Part model, mm, in its own coordinate system. A direction names the side the tool comes from. Give positions to 0.01 mm unless a question says otherwise; leave off trailing zeros. Order: outer loops, then holes, each group sorted by start corner. A loop starts at its lowest first (then second) coordinate and runs counter-clockwise, first axis right, second up. Notation, with made-up numbers: M 1,-6 L 32,-6 A17 ccw 32,-1 Z; hole C -14.75,3.25 d2. An arc over 180 degrees is marked long. Write each question's results on one line, items separated by ' | '. Start each with the question number.
from build123d import *

# Parameters (mm, degrees)
F1_DEPTH = 2540


with BuildPart() as f1:
    # F0 (on Front) → F1 (new body)
    with BuildSketch(Plane.XZ):
        with BuildLine():
            Line((153.9936810732, 85.9075784683), (30.2082335464, 16.8963483059))
            ThreePointArc((30.2082335464, 16.8963483059), (33.4933271093, 8.7304638603), (34.6124827204, 0))
            ThreePointArc((34.6124827204, 0), (33.5294597887, -8.5906511012), (30.3481664655, -16.6437000769))
            Line((30.3481664655, -16.6437000769), (153.9936810732, -85.7974737883))
            Line((153.9936810732, -85.7974737883), (153.9936810732, 85.9075784683))
        make_face()
        with BuildLine():
            ThreePointArc((30.2082335464, 16.8963483059), (0.1433871846, 34.6121857181), (-30.0672068078, 17.1460501237))
            Line((-30.0672068078, 17.1460501237), (0.2459637966, 0.192178832))
            Line((0.2459637966, 0.192178832), (30.2082335464, 16.8963483059))
        make_face()
        with BuildLine():
            Line((30.3481664655, -16.6437000769), (0.2459637966, 0.192178832))
            Line((0.2459637966, 0.192178832), (-30.2550625521, -16.8123511155))
            ThreePointArc((-30.2550625521, -16.8123511155), (0.0963217415, -34.6123486951), (30.3481664655, -16.6437000769))
        make_face()
        with BuildLine():
            Line((0.2459637966, 0.192178832), (-30.0672068078, 17.1460501237))
            ThreePointArc((-30.0672068078, 17.1460501237), (-34.6119531212, 0.1914711524), (-30.2550625521, -16.8123511155))
            Line((-30.2550625521, -16.8123511155), (0.2459637966, 0.192178832))
        make_face()
        with BuildLine():
            Line((30.2082335464, 16.8963483059), (0.2459637966, 0.192178832))
            Line((0.2459637966, 0.192178832), (30.3481664655, -16.6437000769))
            ThreePointArc((30.3481664655, -16.6437000769), (33.5294597887, -8.5906511012), (34.6124827204, 0))
            ThreePointArc((34.6124827204, 0), (33.4933271093, 8.7304638603), (30.2082335464, 16.8963483059))
        make_face()
        with BuildLine():
            Line((-30.0672068078, 17.1460501237), (-153.9936810732, 86.4569619298))
            Line((-153.9936810732, 86.4569619298), (-153.9936810732, -85.7974737883))
            Line((-153.9936810732, -85.7974737883), (-30.2550625521, -16.8123511155))
            ThreePointArc((-30.2550625521, -16.8123511155), (-34.6119531212, 0.1914711524), (-30.0672068078, 17.1460501237))
        make_face()
    extrude(amount=F1_DEPTH)


solid = f1.part
(1) Saw through at B-B on y = -750. Give the cut face in (x, z).
(2) Saw through at C-C on x = 127.5. Give the cut face in (y, z), plus the area to 3 significant figures.
(3) Tool access for faces 1 (the flat face through (92.967, -1252.22, 51.885)), 2 (the flat face through (-92.991, -1252.22, -51.788)), 3 (the flat face through (-2, 0, 2)): list every direction of +Z, -Z, +X, -X, +Y, -Y with a clear straight run to the whole face (end or side of a thin tool).
(4) Probe L1, parallel to X at y = -421, z = 21; L2, parallel to X at y = -2032.5, z = -24.5; L3, parallel to X at y = -251, z = -41. List the from-to ranges inside material, lowest first.
(5) Drop flat-ended pins along their axis: P1, Ø8, axis at x = 76.5, y = -2120, coming from the -Z side; P2, Ø10, axis at x = 0.5, y = -1103, coming from the +Z side; P3, Ø6, axis at x = -32.5, y = -663.5, coming from the +Z side. Give the stop position or say it passes through.
(6) Saw through at A-A on z = -58. Give the cut face in (x, y), plus the area to 3 significant figures.
(7) Pull direction X, two halves, no side cores. Call faces 4 (the flat face through (153.994, -1252, -1)), 5 (the flat face through (-153.994, -1252, 2)), 6 (the flat face through (-2, -2540, 2)), 7 (the cylindrical face through (0.655, -1252.22, 34.606)): +X half, -X half, draft (parallel to the pull), parting line (faces both ways), or undercut.
Taken from the geometry:
1) outline: M -153.99,-85.8 L -30.26,-16.81 A34.61 ccw 30.35,-16.64 L 153.99,-85.8 L 153.99,85.91 L 30.21,16.9 A34.61 ccw -30.07,17.15 L -153.99,86.46 Z
2) outline: M -2540,-70.98 L 0,-70.98 L 0,71.14 L -2540,71.14 Z | area: 361,000 mm²
3) face 1: +Z, +Y, -Y | face 2: -Z, +Y, -Y | face 3: +Z, -Z, +X, -X, +Y
4) L1: x = -153.99 to -36.96, -27.51 to 27.51, 37.57 to 153.99 | L2: x = -153.99 to -44.04, -24.45 to 24.45, 44.4 to 153.99 | L3: x = -153.99 to -73.64, 73.9 to 153.99
5) P1: stops at z = -44.69 | P2: stops at z = 34.61 | P3: stops at z = 20.18
6) outline: M -153.99,-2540 L -104.13,-2540 L -104.13,0 L -153.99,0 Z; M 104.29,-2540 L 153.99,-2540 L 153.99,0 L 104.29,0 Z | area: 253,000 mm²
7) face 4: +X half | face 5: -X half | face 6: draft | face 7: undercut
